from build123d import *

# Parameters (mm, degrees)
F0_R     = 9
F1_DEPTH = 6
F2_R     = 2.5
F3_DEPTH = 46
F4_R     = 8
F4_R_2   = 2.5
F5_DEPTH = 6
F7_D     = 2.5
F7_DEPTH = 17.5
F7_TIP   = 0.7510757738


with BuildPart() as f1:
    # F0 (on Front) → F1 (new body)
    with BuildSketch(Plane.XZ):
        Circle(F0_R)
    extrude(amount=F1_DEPTH)

    # F2 (on Front) → F3 (join)
    with BuildSketch(Plane.XZ):
        Circle(F2_R)
    extrude(amount=-F3_DEPTH)

    # F4 (on face) → F5 (join)
    with BuildSketch(Plane(origin=(0, 46, 0), x_dir=(-1, 0, 0), z_dir=(0, 1, 0))):
        Circle(F4_R)
        Circle(F4_R_2, mode=Mode.SUBTRACT)
    extrude(amount=-F5_DEPTH)

    # F7
    with Locations(Plane.XZ.offset(6)):
        with Locations((0, 0)):
            Hole(F7_D / 2, depth=F7_DEPTH)
            with Locations((0, 0, -(F7_DEPTH + F7_TIP / 2))):  # 118° drill point
                Cone(0, F7_D / 2, F7_TIP, mode=Mode.SUBTRACT)


solid = f1.part
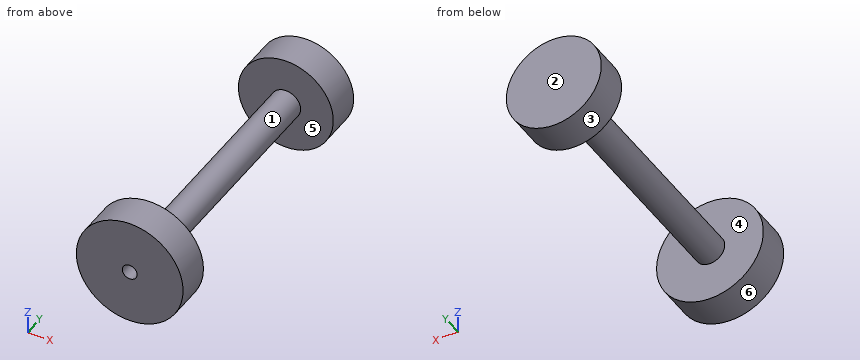
CAD build for the part. Positions are in the model's coordinates, mm. Face numbers are marked on the shaded views. A direction names the side the tool comes from. Round coordinates to 2 decimals unless told otherwise and drop trailing zeros. Write each loop counter-clockwise with the first axis right and the second up, starting at its lowest first coordinate (ties: lowest second). Pieces come first, ordered by that corner, then holes.
(1) Slice it at C-C, the plane y = 34. Write the cut outline in (x, z), and give its area (3 significant figures).
(2) Slice it at A-A, the plane z = -5.75. Write the cut outline in (x, y), and give its area (3 significant figures).
(3) Mould opens along Y. For the marked faces 1, 2, 3 and 4 say: pulls with the +Y half, pulls with the -Y half, needs draft (parallel to the pull), parting line crosses it, or undercut.
(4) Drop flat-ended pins along their axis: P1, Ø1.5, axis at x = -3, y = 38.5, coming from the +Z side; P2, Ø10, axis at y = 28, z = -4.5, coming from the +X side; P3, Ø2, axis at x = 0, z = 0, coming from the -Y side. Give the stop position or say it passes through.
(5) Slice it at B-B, the plane x = 4. Write the cut outline in (y, z).
(6) Probe line 1 along X through (y, z) = (3.25, 0); line 2 along Y through (x, z) = (2, 5.25). List the from-to ranges inside material, lowest first.
(7) 3-axis set-ups, long thin cutter, end or side, ignore diameter. For the marked faces 5 and 6: which of +Z, -Z, +X, -X, +Y, -Y reach the whole face in a straight line?
From the geometry:
1. outline: circle Ø5 at (0, 0)
1. area: 19.6 mm2
2. outline: (-6.92, -6) - (6.92, -6) - (6.92, 0) - (-6.92, 0) - close; (-5.56, 40) - (5.56, 40) - (5.56, 46) - (-5.56, 46) - close
2. area: 150 mm2
3. face 1: undercut
3. face 2: pulls with the +Y half
3. face 3: needs draft
3. face 4: undercut
4. P1: stops at z = 1.09
4. P2: stops at x = 2.5
4. P3: stops at y = 11.65
5. outline: (-6, -8.06) - (0, -8.06) - (0, 8.06) - (-6, 8.06) - close; (40, -6.93) - (46, -6.93) - (46, 6.93) - (40, 6.93) - close
6. line 1: x = -2.5 to -1.25, 1.25 to 2.5
6. line 2: y = -6 to 0, 40 to 46
7. face 5: none
7. face 6: +Y, -Y
